Source: CAD feature listing. Evaluate the final solid. Frame: model axes, mm. Round coordinates to 2 decimals unless told otherwise and drop trailing zeros. Loops run counter-clockwise (first coordinate to the right, second up) from the corner with the lowest first, then second, coordinate; pieces in that order, holes last. Notation, with made-up numbers: M 51,89.25 L 105,89.25 A15 cw 105,117.25 Z; hole C 84.5,-21.5 d5. An arc over 180 degrees is marked long. One line per item, written item: value.
from build123d import *

# Parameters (mm, degrees)
SKETCH1_W           = 4.57
SKETCH1_H           = 143
BOSS_EXTRUDE1_DEPTH = 18
SKETCH2_R           = 2.1
CUT_EXTRUDE1_DEPTH  = 18
SKETCH3_W           = 145
SKETCH3_H           = 3
CUT_EXTRUDE2_DEPTH  = 10


with BuildPart() as part:
    # Sketch1 → Boss-Extrude1 (new body)
    with BuildSketch(Plane(origin=(0, 0, 0), x_dir=(1, 0, 0), z_dir=(0, 1, 0))):
        with Locations((-47.715, 196.5)):
            Rectangle(SKETCH1_W, SKETCH1_H)
    extrude(amount=BOSS_EXTRUDE1_DEPTH)

    # Sketch2 → Cut-Extrude1 (cut)
    with BuildSketch(Plane.ZY.offset(50)):
        with Locations((-127.5, 10.5)):
            Circle(SKETCH2_R)
        with Locations((-140.2, 10.5)):
            Circle(SKETCH2_R)
        with Locations((-152.9, 10.5)):
            Circle(SKETCH2_R)
    extrude(amount=-CUT_EXTRUDE1_DEPTH, mode=Mode.SUBTRACT)

    # Sketch3 → Cut-Extrude2 (cut)
    with BuildSketch(Plane.ZY.offset(50)):
        with Locations((-197.5, 1.5)):
            Rectangle(SKETCH3_W, SKETCH3_H)
    extrude(amount=-CUT_EXTRUDE2_DEPTH, mode=Mode.SUBTRACT)


solid = part.part
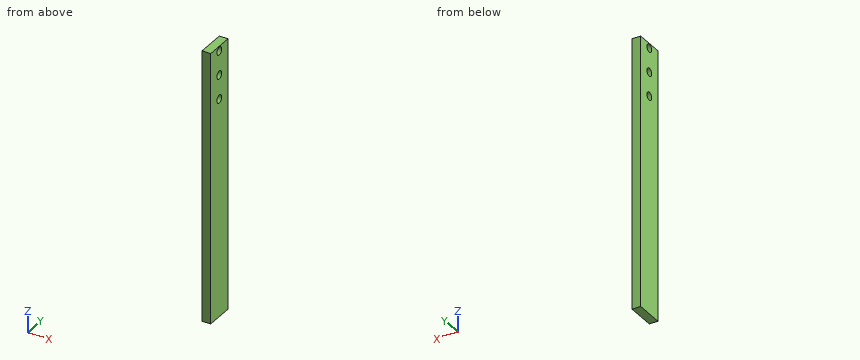
1. Section query B-B (z = -127.5). Return the cut outline in (x, y).
Report:
outline: M -50,3 L -45.43,3 L -45.43,8.4 L -50,8.4 Z; M -50,12.6 L -45.43,12.6 L -45.43,18 L -50,18 Z
2. Section query C-C (x = -46.3). Return the cut outline in (y, z).
Report:
outline: M 3,-268 L 18,-268 L 18,-125 L 3,-125 Z; hole C 10.5,-152.9 d4.2; hole C 10.5,-140.2 d4.2; hole C 10.5,-127.5 d4.2
3. Ray query, line 1 (Y direction, x = -47.55, z = -127.5); line 2 (Z direction, x = -47.1, y = 9.25); line 3 (Z direction, x = -49.45, y = 11). Return the intervals inside material, ascending. Write a range as [from, to].
Report:
line 1: y = [3, 8.4], [12.6, 18]
line 2: z = [-268, -154.59], [-151.21, -141.89], [-138.51, -129.19], [-125.81, -125]
line 3: z = [-268, -154.94], [-150.86, -142.24], [-138.16, -129.54], [-125.46, -125]
4. Section query A-A (y = 10.5). Return the cut outline in (x, z), and give its area (3 significant figures).
Report:
outline: M -50,-268 L -45.43,-268 L -45.43,-155 L -50,-155 Z; M -50,-150.8 L -45.43,-150.8 L -45.43,-142.3 L -50,-142.3 Z; M -50,-138.1 L -45.43,-138.1 L -45.43,-129.6 L -50,-129.6 Z; M -50,-125.4 L -45.43,-125.4 L -45.43,-125 L -50,-125 Z
area: 596 mm2
